Input: part model. Units: mm. Frame: model coordinates. A direction names the side the tool comes from. Round coordinates to 2 decimals unless told otherwise and drop trailing zeros. Loops run counter-clockwise (first coordinate to the right, second up) from the corner with the lowest first, then second, coordinate; pieces in that order, holes last.
1) Access query for faces 1 (the face through (-1, 12.7, -76)), 2 (the face through (94.223, 9.658, 78.264)). Directions: +Z, -Z, +X, -X, +Y, -Y. A direction counts if a zero-diameter tool reaches every point of the face in a straight line with its end or side. Return the directions, or none.
2) Ray query, line 1 along X through (y, z) = (8, -13.5); line 2 along X through (y, z) = (16.25, -72.5); line 3 along Z through (x, y) = (-20.5, 15.25) (3 decimals). Return the intervals inside material, ascending.
3) Section C-C, the plane x = 78. Return loops of the section in (y, z) (3 decimals), and give its area (3 significant figures).
4) First-contact query: pin 1 (5 mm diameter, centred on x = -48.5, z = 27, fed in from +Y); pin 2 (5 mm diameter, centred on x = 74, z = 13, fed in from -Y); pin 3 (3.5 mm diameter, centred on x = 12.5, z = 83.5, fed in from +Y) (3 decimals); pin 4 (6.5 mm diameter, centred on x = -39.5, z = 75, fed in from +Y). Flat tips, straight axial feed; report the tip coordinate or a pass-through.
5) Draft query along Z for faces 3 (the face through (94.256, 9.658, -78.074)), 4 (the face through (-1, 0, -1)), 5 (the face through (-1, 10, 85.725)), 6 (the face through (-1, 3.81, -1)). Return one class per face: pulls with the +Z half, pulls with the -Z half, needs draft (parallel to the pull), parting line crosses it, or undercut.
6) Section B-B, the plane y = 8.75. State how many separate pieces and enclosed holes the cut face has, and give its area (3 significant figures).
7) Section A-A, the plane z = 16. Return loops of the section in (x, y).
from build123d import *

# Parameters (mm, degrees)
SKETCH1_W           = 200.025
SKETCH1_H           = 171.45
BOSS_EXTRUDE1_DEPTH = 19.05
SKETCH2_W           = 193.675
SKETCH2_H           = 139.7
CUT_EXTRUDE1_DEPTH  = 15.24
SKETCH4_W           = 168.275
SKETCH4_H           = 171.45
CUT_EXTRUDE2_DEPTH  = 3.175
SKETCH5_W           = 168.275
SKETCH5_H           = 12.7
CUT_EXTRUDE3_DEPTH  = 3.175
SKETCH7_W           = 168.275
SKETCH7_H           = 12.7
CUT_EXTRUDE5_DEPTH  = 3.175
SKETCH11_R          = 2.2
CUT_EXTRUDE6_DEPTH  = 33.5
FILLET3_R           = 3.81


with BuildPart() as part:
    # Sketch1 → Boss-Extrude1 (new body)
    with BuildSketch(Plane(origin=(0, 0, 0), x_dir=(1, 0, 0), z_dir=(0, 1, 0))):
        Rectangle(SKETCH1_W, SKETCH1_H)
    extrude(amount=BOSS_EXTRUDE1_DEPTH)

    # Sketch2 → Cut-Extrude1 (cut)
    with BuildSketch(Plane(origin=(0, 19.05, 0), x_dir=(1, 0, 0), z_dir=(0, 1, 0))):
        Rectangle(SKETCH2_W, SKETCH2_H)
    extrude(amount=-CUT_EXTRUDE1_DEPTH, mode=Mode.SUBTRACT)

    # Sketch4 → Cut-Extrude2 (cut)
    with BuildSketch(Plane(origin=(0, 19.05, 0), x_dir=(1, 0, 0), z_dir=(0, 1, 0))):
        Rectangle(SKETCH4_W, SKETCH4_H)
    extrude(amount=-CUT_EXTRUDE2_DEPTH, mode=Mode.SUBTRACT)

    # Sketch5 → Cut-Extrude3 (cut)
    with BuildSketch(Plane(origin=(0, 15.875, 0), x_dir=(1, 0, 0), z_dir=(0, 1, 0))):
        with Locations((0, -76.2)):
            Rectangle(SKETCH5_W, SKETCH5_H)
    extrude(amount=-CUT_EXTRUDE3_DEPTH, mode=Mode.SUBTRACT)

    # Sketch7 → Cut-Extrude5 (cut)
    with BuildSketch(Plane(origin=(0, 15.875, 0), x_dir=(1, 0, 0), z_dir=(0, 1, 0))):
        with Locations((0, 76.2)):
            Rectangle(SKETCH7_W, SKETCH7_H)
    extrude(amount=-CUT_EXTRUDE5_DEPTH, mode=Mode.SUBTRACT)

    # Sketch11 → Cut-Extrude6 (cut)
    with BuildSketch(Plane(origin=(0, 19.05, 0), x_dir=(1, 0, 0), z_dir=(0, 1, 0))):
        with Locations(Location((92.075, 77.7875, 0), (0, 0, 270))):
            Circle(SKETCH11_R)
        with Locations(Location((92.075, -77.7875, 0), (0, 0, 90))):
            Circle(SKETCH11_R)
    cut_extrude6 = extrude(amount=-CUT_EXTRUDE6_DEPTH, mode=Mode.SUBTRACT)

    # Fillet3
    fillet3_edges = [part.edges().sort_by_distance(p)[0] for p in [
        (0, 0, 85.725),
        (-100.0125, 0, 0),
        (0, 0, -85.725),
        (100.0125, 0, 0),
        (100.0125, 9.525, 85.725),
        (-100.0125, 9.525, 85.725),
        (-100.0125, 9.525, -85.725),
        (100.0125, 9.525, -85.725),
    ]]
    fillet(fillet3_edges, radius=FILLET3_R)

    # Mirror1: Cut-Extrude6 across plane
    add(cut_extrude6.mirror(Plane(origin=(0, 0, 0), x_dir=(0, 0, 1), z_dir=(1, 0, 0))), mode=Mode.SUBTRACT)


solid = part.part
Final values:
1. face 1: +Y
1. face 2: +Y, -Y
2. line 1: x = -100.01 to -96.84, 96.84 to 100.01
2. line 2: x = -100.01 to -84.14, 84.14 to 100.01
2. line 3: z = -85.725 to -82.55, 82.55 to 85.725
3. outline: (0, -81.915) arc R3.81 ccw to (3.81, -85.725) - (15.875, -85.725) - (15.875, -82.55) - (12.7, -82.55) - (12.7, -69.85) - (3.81, -69.85) - (3.81, 69.85) - (12.7, 69.85) - (12.7, 82.55) - (15.875, 82.55) - (15.875, 85.725) - (3.81, 85.725) arc R3.81 ccw to (0, 81.915) - close
3. area: 949 mm2
4. pin 1: stops at y = 3.81
4. pin 2: stops at y = 0
4. pin 3: stops at y = 15.875
4. pin 4: stops at y = 12.7
5. face 3: undercut
5. face 4: needs draft
5. face 5: pulls with the +Z half
5. face 6: undercut
6. separate pieces: 1
6. enclosed holes: 5
6. area: 7,160 mm2
7. outline: (-100.01, 3.81) arc R3.81 ccw to (-96.2, 0) - (96.2, 0) arc R3.81 ccw to (100.01, 3.81) - (100.01, 19.05) - (96.84, 19.05) - (96.84, 3.81) - (-96.84, 3.81) - (-96.84, 19.05) - (-100.01, 19.05) - close
